Autodesk Inventor part; units mm, degrees
ref_plane "YZ Plane" through (0, 0, 0) normal (1, 0, 0) x (0, 1, 0)
ref_plane "XZ Plane" through (0, 0, 0) normal (0, 1, 0) x (-1, 0, 0)
ref_plane "XY Plane" through (0, 0, 0) normal (0, 0, 1) x (1, 0, 0)
sketch "Sketch1" plane through (0, 0, 0) normal (0, 0, 1) x (1, 0, 0)
  line L0 (0, 0) -> (560, 0)
  line L1 (0, 0) -> (-100, 30)
  line L2 (0, 0) -> (104.4031, 0) construction
  line L3 (-100, 30) -> (-100, 67)
  line L4 (-98.4, 67) -> (-98.4, 31.1904)
  line L5 (-98.4, 31.1904) -> (0.2348, 1.6)
  line L6 (0.2348, 1.6) -> (560, 1.6)
  line L7 (-98.4, 67) -> (-100, 67)
  line L8 (560, 1.6) -> (560, 0)
  dimension "d0" = 560
  dimension "d2" = 100
  dimension "d3" = 37
  dimension "d9" = 30
  dimension "d10" = 1.6
extrude "Extrusion1" add sketch "Sketch1" along normal blind 1900
sketch "Sketch2" plane through (0, 0, 1900) normal (0, 0, 1) x (1, 0, 0)
  line L0 (-98.4, 31.1904) -> (-98.4, 67)
  line L1 (0.2348, 1.6) -> (-98.4, 31.1904)
  line L2 (560, 1.6) -> (0.2348, 1.6)
  line L3 (-78.4, 67) -> (-78.4, 46.0711)
  line L4 (-78.4, 46.0711) -> (3.1702, 21.6)
  line L5 (3.1702, 21.6) -> (560, 21.6)
  line L6 (-78.4, 67) -> (-98.4, 67)
  line L7 (560, 21.6) -> (560, 1.6)
  line L8 (560, 1.6) -> (558.4, 1.6)
  line L9 (558.4, 1.6) -> (558.4, 21.6)
  line L10 (558.4, 21.6) -> (560, 21.6)
  line L11 (560, 21.6) -> (560, 1.6)
  point P0 (0, 0)
  dimension "d11" = 20
  dimension "d16" = 1.6
  dimension "d17" = 20
extrude "Extrusion2" add sketch "Sketch2" against normal blind 1.6
sketch "Sketch3" plane through (0, 0, 0) normal (0, 0, -1) x (-1, 0, 0)
  line L0 (98.4, 67) -> (98.4, 31.1904)
  line L1 (98.4, 67) -> (78.4, 67)
  line L2 (78.4, 67) -> (78.4, 46.0711)
  line L3 (78.4, 46.0711) -> (-3.1702, 21.6)
  line L4 (-3.1702, 21.6) -> (-560, 21.6)
  line L5 (-560, 21.6) -> (-560, 1.6)
  line L6 (-0.2348, 1.6) -> (-560, 1.6)
  line L7 (98.4, 31.1904) -> (-0.2348, 1.6)
  point P0 (0, 0)
extrude "Extrusion3" add sketch "Sketch3" against normal blind 1.6
sketch "Sketch4" plane through (0, 0, 1898.4) normal (0, 0, -1) x (-1, 0, 0)
  line L0 (-560, 21.6) -> (-560, 1.6)
  line L1 (-560, 21.6) -> (-558.4, 21.6)
  line L2 (-558.4, 21.6) -> (-558.4, 1.6)
  line L3 (-558.4, 1.6) -> (-560, 1.6)
  line L4 (-560, 1.6) -> (-560, 21.6)
  point P0 (0, 0)
  dimension "d18" = 1.6
  dimension "d19" = 20
extrude "Extrusion4" add sketch "Sketch4" along normal up to surface (1898.4 mm away)
sketch "Sketch5" plane through (0, 0, 0) normal (0, -1, 0) x (1, 0, 0)
  line L0 (146.0887, 600) -> (346.0887, 600)
  line L1 (346.0887, 600) -> (346.0887, 1300)
  line L2 (346.0887, 1300) -> (146.0887, 1300)
  line L3 (146.0887, 1300) -> (146.0887, 600)
  line L4 (0, 0) -> (560, 0)
  dimension "d22" = 200
  dimension "d23" = 700
  dimension "d24" = 600
extrude "Extrusion5" cut sketch "Sketch5" against normal blind 10
properties part number "Cover Lower Front" material "Steel"
Work out the finished part from the listing and answer in its coordinate system (mm). A direction names the side the tool comes from. Give positions to 0.01 mm unless a question says otherwise; leave off trailing zeros. Write each loop counter-clockwise with the first axis right and the second up, starting at its lowest first coordinate (ties: lowest second). Pieces come first, ordered by that corner, then holes.
Q1. Straight lines are drawn through the part: L1, parallel to Z at x = 459, y = 15; L2, parallel to Y at x = 37.5, z = 1600.5; L3, parallel to X at y = 46.5, z = 1731.5. For each, find the intervals that lie inside material, in ascending order.
Answer:
L1: z = 0 to 1.6, 1898.4 to 1900
L2: y = 0 to 1.6
L3: x = -100 to -98.4
Q2. The part is cut by section D-D on z = 249. Give the vertices of the cut face in (x, y).
Answer:
outline: (-100, 30) - (0, 0) - (560, 0) - (560, 21.6) - (558.4, 21.6) - (558.4, 1.6) - (0.23, 1.6) - (-98.4, 31.19) - (-98.4, 67) - (-100, 67) - close
Q3. The part is cut by section A-A on x = 318.5. Give the vertices of the cut face in (y, z), and give its area (3 significant figures).
Answer:
outline: (0, 0) - (21.6, 0) - (21.6, 1.6) - (1.6, 1.6) - (1.6, 600) - (0, 600) - close; (0, 1300) - (1.6, 1300) - (1.6, 1898.4) - (21.6, 1898.4) - (21.6, 1900) - (0, 1900) - close
area: 1,980 mm2
Q4. For a pull along X with two mould halves and no side action, classify faces 1 (the face through (207, 15, 1.6)), 2 (the face through (-98.4, 49, 937)), 3 (the face through (232, 11, 0)) as released by +X, released by -X, zero draft, split by the parting line, or undercut.
Answer:
face 1: undercut
face 2: released by +X
face 3: zero draft
Q5. A tool of negligible diameter and unlimited length cuts with its end or side. For faces 4 (the face through (228, 11, 1900)), 5 (the face through (-49.77, 16.6, 936.72)), from which of +Z, -Z, +X, -X, +Y, -Y can it reach the whole face along a straight path? Write none if from no direction.
Answer:
face 4: +Z, +X, -X, +Y, -Y
face 5: +Y
Q6. The part is cut by section B-B on z = 682.5. Give the vertices of the cut face in (x, y).
Answer:
outline: (-100, 30) - (0, 0) - (146.09, 0) - (146.09, 1.6) - (0.23, 1.6) - (-98.4, 31.19) - (-98.4, 67) - (-100, 67) - close; (346.09, 0) - (560, 0) - (560, 21.6) - (558.4, 21.6) - (558.4, 1.6) - (346.09, 1.6) - close
Q7. Given pin 1 (0.5 mm diameter, centred on y = 61, z = 1899.5, fed in from +X); pin 2 (6 mm diameter, centred on y = 57.5, z = 1529.5, fed in from +X); pin 3 (10 mm diameter, centred on x = 240, z = 1366.5, fed in from -Y); pin 4 (1 mm diameter, centred on x = 277.5, z = 414.5, fed in from +Y), each flat-ended and moving along its own axis, determine where each tip first touches the part or whether it passes through.
Answer:
pin 1: stops at x = -78.4
pin 2: stops at x = -98.4
pin 3: stops at y = 0
pin 4: stops at y = 1.6
Q8. The part is cut by section C-C on y = 56.5. Give the vertices of the cut face in (x, z).
Answer:
outline: (-100, 0) - (-78.4, 0) - (-78.4, 1.6) - (-98.4, 1.6) - (-98.4, 1898.4) - (-78.4, 1898.4) - (-78.4, 1900) - (-100, 1900) - close
